For this review, take the finished solid that the model builds, in its own axes (mm). A direction names the side the tool comes from. Give positions to 0.01 mm unless a question says otherwise; leave off trailing zeros. One line per question, with ' | ' between items. Start each with the question number.
(1) Wall thickness on probe 1 along X at (y, z) = (-10, 0) (1 decimal); probe 2 along Y at (x, z) = (11, 0) (3 decimals): over which ranges is each line inside the solid? List them lowest first.
(2) Tool access review of faces 5 (the cylindrical face through (2, 4, 0)), 6 (the flat face through (15.6, -4, 0)), 7 (the cylindrical face through (8.61, -3.1, 0.69)), 8 (the cylindrical face through (-1.514, -12.694, 0.477)): name each direction out of +Z, -Z, +X, -X, +Y, -Y from which nothing blocks a thin tool from reaching the whole face with its end or side.
(3) Insertion check: P1, Ø1, axis at x = 13, z = -1, coming from the -Y side; P2, Ø1.5, axis at y = -10.5, z = 3, coming from the -X side; P3, Ø5, axis at y = 1, z = -0.5, coming from the +X side. Each pin has a flat end and moves straight along its axis. Give the tip position at first contact, or say it passes through.
(4) Draft analysis for pull direction X (two halves, no side actions). For faces 1 (the conical face through (3.69, 4.05, 1.28)), 2 (the flat face through (-2, -22.8, 0)), 3 (the cylindrical face through (0.95, -13.94, 3.03)), 4 (the flat face through (13.2, 4, -1)), state which applies: +X half, -X half, draft (parallel to the pull), parting line (faces both ways), or undercut.
from build123d import *

# Parameters (mm, degrees)
SKETCH1_R             = 4
BASE_EXTRUDE_DEPTH    = 3.6
RBODY_SKETCH_R        = 5.55
RBODY_DEPTH           = 9.6
ELBOW_ANGLE           = 90
SKETCH3_R             = 4
BOSS_EXTRUDE1_DEPTH   = 5.6
STEM_SKETCH_R         = 3.175
STEM_DEPTH            = 17.2
RTUBE_START           = -13.3
RTUBE_SKETCH_R        = 3.175
RTUBE_DEPTH           = 13.3
RTUBE_RADIUS_R        = 0.5
DIAMETER_R            = 1.5875
PORT_THREADS_REACH    = 34.831
PORT_THREADS_SKETCH_R = 1.5875


with BuildPart() as part:
    # Sketch1 → Base-Extrude (new body)
    with BuildSketch(Plane(origin=(0, 0, 0), x_dir=(0, 0, -1), z_dir=(1, 0, 0))):
        with Locations(Location((0, 0, 0), (0, 0, 180))):
            Circle(SKETCH1_R)
    extrude(amount=BASE_EXTRUDE_DEPTH)

    # RBody_Sketch → RBody (add)
    with BuildSketch(Plane(origin=(3.6, 0, 0), x_dir=(0, 0, -1), z_dir=(1, 0, 0))):
        Circle(RBODY_SKETCH_R)
    extrude(amount=RBODY_DEPTH)

    # RBody_Chamfer: read off the stored shape, not the designer's step
    # RBody_Chamfer outline → RBody_Chamfer (revolve, cut)
    with BuildSketch(Plane.YX):
        Polygon((5.55, 4.164153863), (4, 3.6), (5.55, 3.6), align=None)
    revolve(axis=Axis((0, 0, 0), (1, 0, 0)), mode=Mode.SUBTRACT)

    # RRelease_Sketch → RRelease (revolve)
    with BuildSketch(Plane.XY, mode=Mode.PRIVATE) as rrelease_sk:
        with BuildLine():
            Line((13.2, 3.925), (14.1, 3.925))
            Line((14.1, 3.925), (14.1, 5.025))
            Line((14.1, 5.025), (15.1, 5.025))
            ThreePointArc((15.1, 5.025), (15.453553391, 4.878553391), (15.6, 4.525))
            Line((15.6, 4.525), (15.6, 0))
            Line((15.6, 0), (13.2, 0))
            Line((13.2, 0), (13.2, 3.925))
        make_face()
    revolve(rrelease_sk.sketch.rotate(Axis((12.597722381, 0, 0), (1, 0, 0)), 90), axis=Axis((12.597722381, 0, 0), (1, 0, 0)))

    # Elbow_Sketch → Elbow (revolve)
    with BuildSketch(Plane.ZY):
        with BuildLine():
            Line((-4, 0), (4, 0))
            ThreePointArc((4, 0), (0, 4), (-4, 0))
        make_face()
    revolve(axis=Axis((0, 0, -6.487672297), (0, 0, 1)), revolution_arc=ELBOW_ANGLE)

    # Sketch3 → Boss-Extrude1 (add)
    with BuildSketch(Plane.XZ):
        with Locations(Location((0, 0, 0), (0, 0, 90))):
            Circle(SKETCH3_R)
    extrude(amount=BOSS_EXTRUDE1_DEPTH)

    # Stem_Sketch → Stem (add)
    with BuildSketch(Plane(origin=(0, -5.6, 0), x_dir=(-1, 0, 0), z_dir=(0, 1, 0))):
        with Locations(Location((0, 0, 0), (0, 0, 90))):
            Circle(STEM_SKETCH_R)
    extrude(amount=-STEM_DEPTH)

    # RTube_Sketch → RTube (cut)
    with BuildSketch(Plane(origin=(15.6, 0, 0), x_dir=(0, 0, -1), z_dir=(1, 0, 0)).offset(RTUBE_START)):
        Circle(RTUBE_SKETCH_R)
    extrude(amount=RTUBE_DEPTH, mode=Mode.SUBTRACT)

    # RTube_Radius
    rtube_radius_edges = [part.edges().sort_by_distance(p)[0] for p in [
        (15.6, 0, 3.175),
    ]]
    fillet(rtube_radius_edges, radius=RTUBE_RADIUS_R)

    # Stem_Chamfer: read off the stored shape, not the designer's step
    # Stem_Chamfer outline → Stem_Chamfer (revolve, cut)
    with BuildSketch(Plane.XY):
        Polygon((3.175, -22.511324865), (2.675, -22.8), (3.175, -22.8), align=None)
    revolve(axis=Axis((0, 0, 0), (0, 1, 0)), mode=Mode.SUBTRACT)

    # Port_Curve: sweep along a path in Profile
    with BuildLine(Plane.XY) as port_curve_path:
        ThreePointArc((2.3, 0), (0.673654403, -0.673654403), (0, -2.3))
    # Diameter → Port_Curve (sweep, cut)
    with BuildSketch(Plane(origin=(2.3, 0, 0), x_dir=(0, 0, -1), z_dir=(1, 0, 0))):
        Circle(DIAMETER_R)
    sweep(path=port_curve_path.line, mode=Mode.SUBTRACT)

    # Port_Threads_Sketch → Port_Threads (cut, up to next)
    with BuildSketch(Plane(origin=(0, -22.8, 0), x_dir=(-1, 0, 0), z_dir=(0, 1, 0)), mode=Mode.PRIVATE) as port_threads_sk1:
        Circle(PORT_THREADS_SKETCH_R)
    port_threads_tool1 = extrude(port_threads_sk1.sketch, amount=PORT_THREADS_REACH, mode=Mode.PRIVATE) & part.part
    add(port_threads_tool1.solids().sort_by_distance((0, -22.8, 0))[0], mode=Mode.SUBTRACT)


solid = part.part
A:
1) probe 1: x = -3.2 to -1.6, 1.6 to 3.2 | probe 2: y = -5.55 to -3.175, 3.175 to 5.55
2) face 5: none | face 6: +Z, -Z, +X, +Y, -Y | face 7: +X | face 8: -Y
3) P1: stops at y = -5.53 | P2: stops at x = -2.24 | P3: stops at x = 15.6
4) face 1: undercut | face 2: draft | face 3: parting line | face 4: undercut
